Part print with two shaded views. Sizes in mm from the minimum x, y, z corner. A direction names the side the tool comes from. Round coordinates to 2 decimals unless told otherwise and drop trailing zeros. Order: outer loops, then holes, each group sorted by start corner. A loop starts at its lowest first (then second) coordinate and runs counter-clockwise, first axis right, second up. Notation, with made-up numbers: (40, -13.5) - (87, -13.5) arc R14 ccw to (87, 0.5) - close; hole circle Ø5 at (-13, 42). An arc over 180 degrees is marked (long way). Write item = value, one per line.
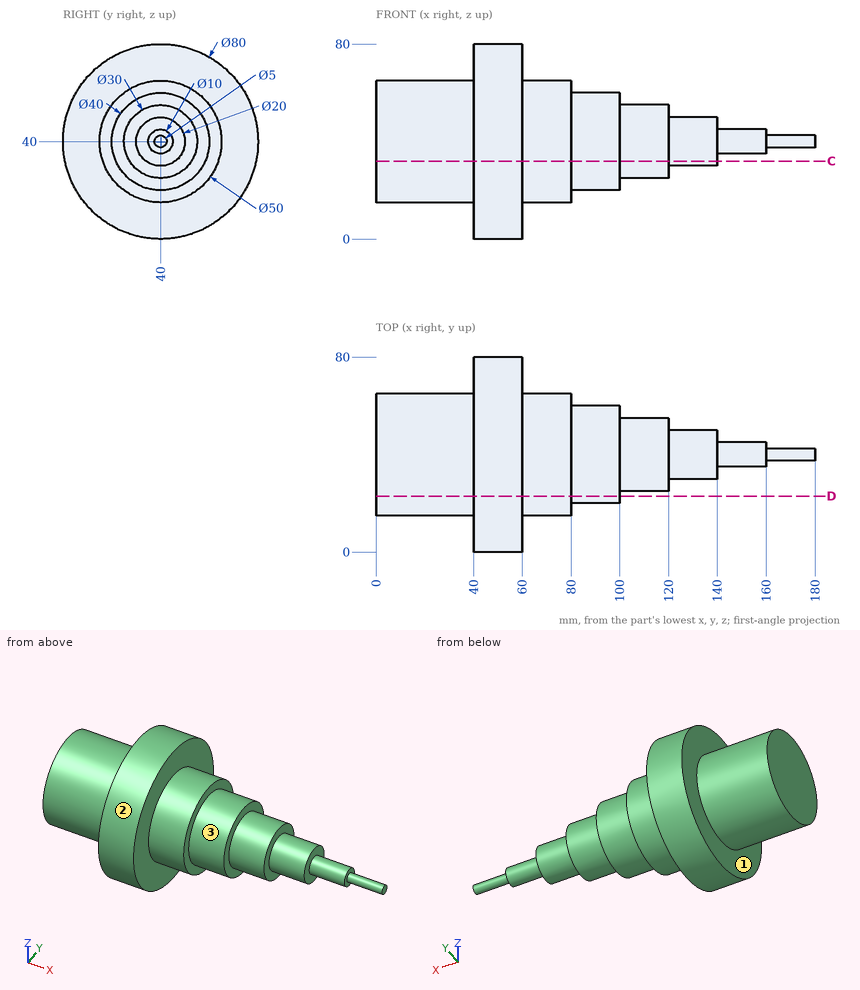
1) Flat gauge pins, fed straight in: pin 1 Ø8 at (x, z) = (45, 63) entering from +Y; pin 2 Ø3 at (x, z) = (25, 48) entering from -Y; pin 3 Ø6 at (x, z) = (108.5, 39.5) entering from +Y. Where does each tip first touch, or does it go through?
Conclusion:
pin_1 = 75.2
pin_2 = 15.86
pin_3 = 55
2) Wall check: line 1 along X through (y, z) = (36.5, 6.5); line 2 along Z through (x, y) = (79.5, 20); line 3 along X through (y, z) = (52, 53). Give the ranges that are in metal, low to high.
Conclusion:
line_1 = 40 to 60
line_2 = 25 to 55
line_3 = 0 to 100
3) 3-axis set-ups, long thin cutter, end or side, ignore diameter. For the marked faces 1, 2 and 3: which of +Z, -Z, +X, -X, +Y, -Y reach the whole face in a straight line?
Conclusion:
face_1 = -X
face_2 = +X, -X
face_3 = +X
4) Cut at D-D (y = 23). Write the cut outline in (x, z), and give its area (3 significant figures).
Conclusion:
outline = (0, 21.67) - (40, 21.67) - (40, 3.79) - (60, 3.79) - (60, 21.67) - (80, 21.67) - (80, 29.46) - (100, 29.46) - (100, 50.54) - (80, 50.54) - (80, 58.33) - (60, 58.33) - (60, 76.21) - (40, 76.21) - (40, 58.33) - (0, 58.33) - close
area = 4,070 mm^2
5) Cut at C-C (z = 32). Write the cut outline in (x, y), and give its area (3 significant figures).
Conclusion:
outline = (0, 16.31) - (40, 16.31) - (40, 0.81) - (60, 0.81) - (60, 16.31) - (80, 16.31) - (80, 21.67) - (100, 21.67) - (100, 27.31) - (120, 27.31) - (120, 34) - (140, 34) - (140, 46) - (120, 46) - (120, 52.69) - (100, 52.69) - (100, 58.33) - (80, 58.33) - (80, 63.69) - (60, 63.69) - (60, 79.19) - (40, 79.19) - (40, 63.69) - (0, 63.69) - close
area = 5,890 mm^2
